For this review, take the finished solid that the model builds, in its own axes (mm). A direction names the side the tool comes from. Round coordinates to 2 decimals unless told otherwise and drop trailing zeros. Order: outer loops, then holes, each group sorted by start corner. A loop starts at its lowest first (then second) coordinate and runs counter-clockwise, first axis right, second up. Notation, with made-up numbers: M -31,-21 L 18,-21 A15 ccw 18,4 Z; hole C 73,-39.75 d11. An arc over 180 degrees is marked long. Answer in a Markdown table with one row per item. Add a question column.
Autodesk Inventor part; units mm, degrees
ref_plane "YZ Plane" through (0, 0, 0) normal (1, 0, 0) x (0, 1, 0)
ref_plane "XZ Plane" through (0, 0, 0) normal (0, 1, 0) x (-1, 0, 0)
ref_plane "XY Plane" through (0, 0, 0) normal (0, 0, 1) x (1, 0, 0)
sketch "Sketch1" plane through (0, 0, 0) normal (0, 1, 0) x (-1, 0, 0)
  line L0 (-27.0524, -30.5) -> (0, -30.5)
  line L1 (-27.0524, -30.5) -> (-27.0524, 0)
  line L2 (-27.0524, 0) -> (0, 0)
  line L3 (0, 0) -> (0, -30.5)
  point P0 (-13.5262, -30.5)
extrude "Extrusion1" add sketch "Sketch1" along normal blind 1.5
sketch "Sketch2" plane through (0, 0, 0) normal (0, -1, 0) x (1, 0, 0)
  circle A0 centre (2.2262, -20) radius 2.2262
  circle A1 centre (24.8262, -20) radius 2.2262
  point P0 (0, 0)
  point P1 (13.5262, -30.5)
  point P2 (27.0524, -30.5)
extrude "Extrusion2" add sketch "Sketch2" against normal blind 3.4
sketch "Sketch3" plane through (0, 0, 0) normal (0, -1, 0) x (1, 0, 0)
  circle A0 centre (24.8262, -19.9938) radius 1.016
  circle A1 centre (2.2262, -20) radius 1.016
  point P0 (0, 0)
  point P1 (13.5262, 0)
  point P2 (1.4262, -20)
  point P3 (0, -30.5)
  dimension "d4" = 2.032
extrude "Extrusion3" cut sketch "Sketch3" against normal up to surface (3.4 mm away)
sketch "Sketch4" plane through (0, 0, 0) normal (0, -1, 0) x (1, 0, 0)
  circle A0 centre (24.8262, -19.9938) radius 2.032
  circle A1 centre (2.2262, -20) radius 2.032
  line L0 (2.2262, -20) -> (0, -20)
  line L1 (0, -20) -> (0, -30.5)
  line L2 (0, -30.5) -> (0, 0)
  point P0 (13.5262, 0)
  dimension "d7" = 4.064
  dimension "d8" = 4.064
extrude "Extrusion4" cut sketch "Sketch4" against normal blind 2.051
sketch "Sketch13" plane through (0, 1.5, 0) normal (0, 1, 0) x (1, 0, 0)
  arc A0 (22.0156, 32.63) -> (24.5977, 30.5) centre (24.5977, 33.13) ccw
  arc A1 (2.4547, 30.5) -> (5.0367, 32.63) centre (2.4547, 33.13) ccw
  line L0 (22.0156, 32.63) -> (5.0367, 32.63)
  arc A2 (2.4547, 30.5) -> (5.0367, 32.63) centre (2.4547, 33.13) ccw
  line L1 (27.0524, 20) -> (27.0524, 30.5)
  line L2 (2.4547, 30.5) -> (24.5977, 30.5)
  line L3 (27.0524, 30.5) -> (0, 30.5)
  point P0 (0, 0)
  point P1 (13.5262, 31)
  point P2 (24.5977, 30.5)
extrude "Extrusion11" add sketch "Sketch13" against normal up to surface (1.5 mm away)
sketch "Sketch14" plane through (0, 1.5, 0) normal (0, 1, 0) x (1, 0, 0)
  line L0 (27.0478, 29.5) -> (21.7177, 29.5)
  line L1 (21.7177, 31.63) -> (5.3347, 31.63)
  line L2 (21.7177, 31.63) -> (21.7177, 29.5)
  line L3 (21.7177, 31.63) -> (5.3347, 31.63)
  line L4 (5.3347, 31.63) -> (5.3347, 29.5)
  line L5 (0, 29.5) -> (4.5847, 29.5)
  line L6 (5.3347, 29.5) -> (4.5847, 29.5)
  line L7 (4.5847, 29.5) -> (0, 29.5)
  line L8 (2.4547, 30.5) -> (0, 30.5)
  line L9 (0, 29.5) -> (0, 30.5)
  line L10 (0, 30.5) -> (2.4547, 30.5)
  arc A0 (2.4547, 30.5) -> (5.0367, 32.63) centre (2.4547, 33.13) ccw
  line L11 (5.0367, 32.63) -> (22.0156, 32.63)
  line L12 (5.0367, 32.63) -> (22.0156, 32.63)
  line L13 (27.0524, 30.5) -> (27.0524, 29.5)
  line L14 (27.0524, 29.5) -> (27.0524, 30.5)
  line L15 (27.0524, 30.5) -> (24.5977, 30.5)
  arc A1 (22.0156, 32.63) -> (24.5977, 30.5) centre (24.5977, 33.13) ccw
  arc A2 (22.0156, 32.63) -> (24.5977, 30.5) centre (24.5977, 33.13) ccw
  arc A3 (2.4547, 30.5) -> (5.0367, 32.63) centre (2.4547, 33.13) ccw
  line L16 (27.0524, 30.5) -> (24.5977, 30.5)
  line L17 (0, 29.5) -> (5.3347, 29.5)
  line L18 (5.3347, 31.63) -> (5.3347, 29.5)
  line L19 (5.3347, 31.63) -> (21.7177, 31.63)
  line L20 (21.7177, 29.5) -> (21.7177, 31.63)
  line L21 (21.7177, 29.5) -> (27.0524, 29.5)
  line L22 (27.0524, 0) -> (27.0524, 30.5)
  line L23 (27.0524, 29.5) -> (27.0524, 30.5)
  arc A4 (22.0156, 32.63) -> (24.5977, 30.5) centre (24.5977, 33.13) ccw
  line L24 (27.0524, 30.5) -> (24.5977, 30.5)
  line L25 (22.0156, 32.63) -> (5.0367, 32.63)
  line L26 (22.0156, 32.63) -> (5.0367, 32.63)
  line L27 (2.4547, 30.5) -> (0, 30.5)
  line L28 (2.4547, 30.5) -> (0, 30.5)
  line L29 (0, 30.5) -> (0, 29.5)
  arc A5 (2.4547, 30.5) -> (5.0367, 32.63) centre (2.4547, 33.13) ccw
  arc A6 (22.0156, 32.63) -> (24.5977, 30.5) centre (24.5977, 33.13) ccw
  point P0 (0, 0)
  point P1 (13.5262, 31)
extrude "Extrusion12" cut sketch "Sketch14" against normal blind 0.5
properties part number "ExpansionCard_SelfTapping_Lid"
1. Consider section B-B on y = 2.9. Write out the cut boundary in (x, z), plus the area to 3 significant figures.
2. Clearance check with flat-ended pins moving along their axes: pin 1 Ø0.9 at (x, z) = (18.5, -32) entering from +Y; pin 2 Ø1.1 at (x, y) = (1.5, 0.5) entering from -Z; pin 3 Ø3.5 at (x, z) = (24.83, -19.99) entering from -Y. State where each tip first meets the part, or that it passes through.
3. Consider section A-A on x = 13. Write out the cut boundary in (y, z), plus the area to 3 significant figures.
4. For faces 5 (the cylindrical face through (26.95, 2.44, -19.33)), 6 (the flat face through (25.8, 0.5, -30.5)), 7 (the flat face through (1, 2.051, -20)), 8 (the flat face through (1.2, 0.5, -30.5)), list the 3-axis set-ups (+Z, -Z, +X, -X, +Y, -Y) from which the entire face can be reached by the end or side of a thin tool; tool diameter is ignored.
5. To check wall thickness, follow probe 1 along X at (y, z) = (0.75, -20); probe 2 along X at (y, z) = (0.35, -21); probe 3 along Y at (x, z) = (17.75, -2). State the ranges of each line that lie inside material, in increasing order. Write a range as [from, to].
6. The part is to be moulded in two halves that separate along X. For faces 1 (the cylindrical face through (22.9, 0.51, -31.12)), 2 (the flat face through (24, 2.051, -19)), 3 (the flat face through (14, 1, 0)), 4 (the flat face through (0, 1, -15)), say which applies: pulls with the +X half, pulls with the -X half, needs draft (parallel to the pull), parting line crosses it, or undercut.
7. Consider section D-D on x = 3.75. Write out the cut boundary in (y, z), plus the area to 3 significant figures.
8. Consider section C-C on z = -25. Write out the cut boundary in (x, y).
Solved:
| question | item | result |
|---|---|---|
| 1 | outline | C 2.23,-20 d4.45; C 24.83,-20 d4.45; hole C 2.23,-20 d2.03; hole C 24.83,-19.99 d2.03 |
| 1 | area | 24.7 mm^2 |
| 2 | pin 1 | stops at y = 1.5 |
| 2 | pin 2 | stops at z = -30.5 |
| 2 | pin 3 | stops at y = 2.05 |
| 3 | outline | M 0,-32.63 L 1,-32.63 L 1,-31.63 L 1.5,-31.63 L 1.5,0 L 0,0 Z |
| 3 | area | 48.4 mm^2 |
| 4 | face 5 | +Y |
| 4 | face 6 | -Z, +X, +Y, -Y |
| 4 | face 7 | -Y |
| 4 | face 8 | -Z, -X, +Y, -Y |
| 5 | probe 1 | x = [0, 0.19], [4.26, 22.79], [26.86, 27.05] |
| 5 | probe 2 | x = [0, 0.46], [4, 23.06], [26.59, 27.05] |
| 5 | probe 3 | y = [0, 1.5] |
| 6 | face 1 | pulls with the +X half |
| 6 | face 2 | undercut |
| 6 | face 3 | needs draft |
| 6 | face 4 | pulls with the -X half |
| 7 | outline | M 0,-30.84 L 1,-30.84 L 1,-29.5 L 1.5,-29.5 L 1.5,-21.62 L 3.4,-21.62 L 3.4,-18.38 L 1.5,-18.38 L 1.5,0 L 0,0 L 0,-18.66 L 2.05,-18.66 L 2.05,-21.34 L 0,-21.34 Z |
| 7 | area | 46.2 mm^2 |
| 8 | outline | M 0,0 L 27.05,0 L 27.05,1.5 L 0,1.5 Z |
